Geometry: see drawing. Coordinates: mm, zero at the bounding-box minimum. Round coordinates to 2 decimals unless told otherwise and drop trailing zeros. Write each loop counter-clockwise with the first axis right and the second up, starting at its lowest first coordinate (ties: lowest second). Pieces come first, ordered by that corner, then holes. Notation, with made-up numbers: (62.5, 49.25) -> (68.5, 49.25) arc R9 cw to (68.5, 65.25) -> close; hole circle Ø2 at (-15.75, 29.25). An arc over 180 degrees is marked (long way). Write item = value, one per line.
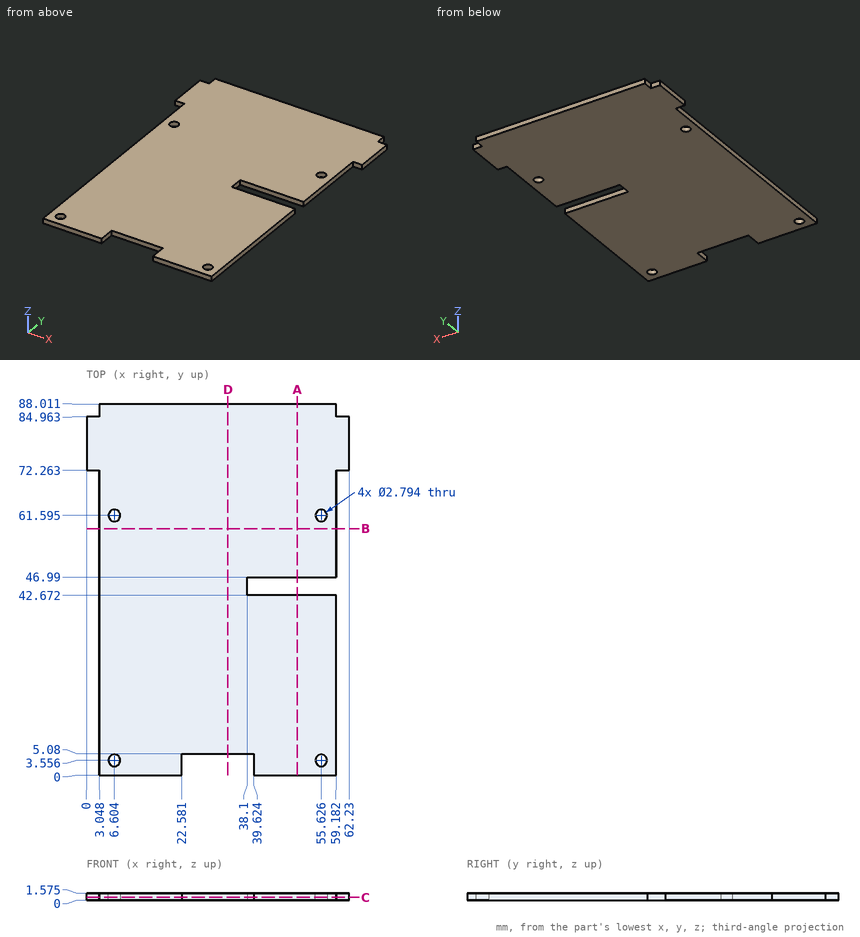
1) Cut plane B-B (y = 58.5). Return the cut outline in (x, z) (1 decimal).
Solutions:
outline = (3, 0) -> (59.2, 0) -> (59.2, 1.6) -> (3, 1.6) -> close
2) First-contact query: P1, Ø3, axis at x = 6.604, y = 61.595, coming from the -Z side; P2, Ø0.5, axis at x = 61, z = 1, coming from the +Y side; P3, Ø0.8, axis at y = 45, z = 0.5, coming from the +X side; P4, Ø0.8, axis at y = 13.5, z = 1, coming from the +X side. Flat tips, straight axial feed; report the tip coordinate or a pass-through.
Solutions:
P1 = 0
P2 = 84.96
P3 = 38.1
P4 = 59.18
3) Cut plane C-C (z = 0.65). Return the cut outline in (x, y) (1 decimal), and give its area (3 significant figures).
Solutions:
outline = (0, 72.3) -> (3, 72.3) -> (3, 0) -> (22.6, 0) -> (22.6, 5.1) -> (39.6, 5.1) -> (39.6, 0) -> (59.2, 0) -> (59.2, 42.7) -> (38.1, 42.7) -> (38.1, 47) -> (59.2, 47) -> (59.2, 72.3) -> (62.2, 72.3) -> (62.2, 85) -> (59.2, 85) -> (59.2, 88) -> (3, 88) -> (3, 85) -> (0, 85) -> close; hole circle Ø2.8 at (6.6, 3.6); hole circle Ø2.8 at (6.6, 61.6); hole circle Ø2.8 at (55.6, 3.6); hole circle Ø2.8 at (55.6, 61.6)
area = 4,820 mm^2
4) Line query: L1, parallel to Y at x = 49, z = 1.35; L2, parallel to Y at x = 7.5, z = 0.65 (1 decimal); L3, parallel to X at y = 20, z = 1.3. Output: solid intervals per line, ascending. Write a range as from..to.
Solutions:
L1 = 0..42.67, 46.99..88.01
L2 = 0..2.5, 4.6..60.5, 62.7..88
L3 = 3.05..59.18
5) Cut plane A-A (x = 50). Return the cut outline in (y, z) (1 decimal), and give its area (3 significant figures).
Solutions:
outline = (0, 0) -> (42.7, 0) -> (42.7, 1.6) -> (0, 1.6) -> close; (47, 0) -> (88, 0) -> (88, 1.6) -> (47, 1.6) -> close
area = 132 mm^2
6) Cut plane D-D (x = 33.5). Return the cut outline in (y, z) (1 decimal).
Solutions:
outline = (5.1, 0) -> (88, 0) -> (88, 1.6) -> (5.1, 1.6) -> close
